Build history of the part. All positions in model axes, mm. Face numbers are marked on the shaded views. Give positions to 0.01 mm unless a question says otherwise; leave off trailing zeros. Order: outer loops, then holes, each group sorted by start corner. A loop starts at its lowest first (then second) coordinate and runs counter-clockwise, first axis right, second up. Notation, with made-up numbers: (46.5, 78) -> (62.5, 78) arc R16 cw to (62.5, 91) -> close; hole circle Ø2 at (26.5, 45). An arc over 180 degrees is marked (long way). One line per item, written item: value. Start each with the question number.
(1) Saw through at A-A on z = -31.75. Give the cut face in (x, y), plus the area to 3 significant figures.
(2) Pin check, flat tips, straight feed: pin 1 (3.5 mm diameter, centred on y = -3.37, z = 65.18, fed in from +X); pin 2 (0.5 mm diameter, centred on x = 1, y = 2, fed in from +Z); pin 3 (7 mm diameter, centred on y = 0, z = 0, fed in from +X); pin 4 (0.8 mm diameter, centred on x = 0.5, z = -20.5, fed in from -Y). Stop position of each tip, or through.
(3) Probe line 1 (Y direction, x = 1.55, z = 67); line 2 (Y direction, x = 0.2, z = -33.5); line 3 (Z direction, x = 0.9, y = 68.5). List the from-to ranges inside material, lowest first.
(4) Saw through at C-C on x = 0.8. Count the separate pieces of the cut face and the enclosed holes in it, plus the area to 3 significant figures.
(5) Two-plate mould, pull along X, no slides. Class the marked faces 1 and 2: +X half, -X half, draft (parallel to the pull), parting line (faces both ways), or undercut.
(6) Saw through at B-B on y = 44.45. Give the cut face in (x, z).
(7) Saw through at D-D on z = 16.5. Give the cut face in (x, y), plus the area to 3 significant figures.
Autodesk Inventor part; units mm, degrees
ref_plane "YZ Plane" through (0, 0, 0) normal (1, 0, 0) x (0, 1, 0)
ref_plane "XZ Plane" through (0, 0, 0) normal (0, 1, 0) x (-1, 0, 0)
ref_plane "XY Plane" through (0, 0, 0) normal (0, 0, 1) x (1, 0, 0)
sketch "main" plane through (0, 0, 0) normal (0, 0, 1) x (1, 0, 0)
  circle A0 centre (-191.7635, 49.9495) radius 2.1844
  circle A1 centre (-95.8324, -13.8772) radius 2.1
  arc A2 (-99.5462, -18.9735) -> (-92.0695, -8.7075) centre (-95.8064, -13.8415) ccw
  arc A3 (-198.1111, 49.7757) -> (-191.7635, 43.5995) centre (-191.7635, 49.9495) ccw
  line L0 (-200.5697, 139.5363) -> (-198.1111, 49.7757)
  arc A4 (-199.0195, 139.7975) -> (-92.0695, -8.7075) centre (80.274, 228.1743) ccw
  circle A5 centre (-195.1368, 115.1254) radius 2.0828
  line L1 (-191.7635, 43.5995) -> (-186.2072, 43.5995)
  arc A6 (-199.0195, 139.7975) -> (-200.5697, 139.5363) centre (-199.7762, 139.5581) ccw
  circle A7 centre (-135.2274, 18.1995) radius 2.0828
  circle A8 centre (-191.7635, 8.6745) radius 2.1844
  arc A9 (-191.7635, 15.0245) -> (-193.2141, 2.4924) centre (-191.7635, 8.6745) ccw
  line L2 (-185.4135, 15.8183) -> (-185.4135, 42.8058)
  line L3 (-191.7635, 15.0245) -> (-186.2072, 15.0245)
  arc A10 (-185.4135, 42.8058) -> (-186.2072, 43.5995) centre (-186.2072, 42.8058) ccw
  arc A11 (-186.2072, 15.0245) -> (-185.4135, 15.8183) centre (-186.2072, 15.8183) ccw
  line L4 (-193.2141, 2.4924) -> (-97.2571, -20.0236)
  point P0 (1.1251, 9.7944)
  point P1 (-200.7302, 145.398)
  dimension "d7" = 12.7
  dimension "d8" = 4.1656
  dimension "d9" = 6.35
  dimension "d11" = 0.7937
  dimension "d13" = 4.1656
  dimension "d15" = 12.7
  dimension "d16" = 0.7937
sketch "Sketch1" plane through (0, 0, 0) normal (1, 0, 0) x (0, 1, 0)
  circle A0 centre (44.45, -15.875) radius 2.0955
  circle A1 centre (0, 0) radius 2.1844
  circle A2 centre (95.9311, -63.8268) radius 2.1
  arc A3 (92.2173, -68.923) -> (99.694, -58.6571) centre (95.9571, -63.7911) ccw
  arc A4 (-6.3476, -0.1739) -> (0, -6.35) centre (0, 0) ccw
  line L0 (-8.8062, 89.5868) -> (-6.3476, -0.1739)
  arc A5 (-7.256, 89.848) -> (99.694, -58.6571) centre (272.0375, 178.2247) ccw
  circle A6 centre (-3.3733, 65.1759) radius 2.0828
  line L1 (0, -6.35) -> (5.5563, -6.35)
  arc A7 (-7.256, 89.848) -> (-8.8062, 89.5868) centre (-8.0127, 89.6085) ccw
  circle A8 centre (56.5361, -31.75) radius 2.0828
  circle A9 centre (0, -41.275) radius 2.1844
  arc A10 (0, -34.925) -> (-1.4506, -47.4571) centre (0, -41.275) ccw
  line L2 (6.35, -34.1313) -> (6.35, -7.1438)
  line L3 (0, -34.925) -> (5.5563, -34.925)
  arc A11 (6.35, -7.1438) -> (5.5563, -6.35) centre (5.5563, -7.1437) ccw
  arc A12 (5.5563, -34.925) -> (6.35, -34.1313) centre (5.5563, -34.1313) ccw
  line L4 (-1.4506, -47.4571) -> (94.5064, -69.9732)
  dimension "d18" = 4.191
extrude "Extrusion1" add sketch "Sketch1" along normal blind 1.5875
equation "\"BendRadius\" = Thickness"
equation "\"BendReliefWidth\" = Thickness"
equation "\"BendReliefDepth\" = 0.5 * Thickness"
equation "\"CornerReliefSize\" = 4 * Thickness"
equation "\"MinimumRemnant\" = 2 * Thickness"
equation "\"TransitionRadius\" = BendRadius"
equation "\"JacobiRadiusSize\" = BendRadius"
equation "\"GapSize\" = Thickness"
properties part number "ramp" material "Acetal Resin, White"
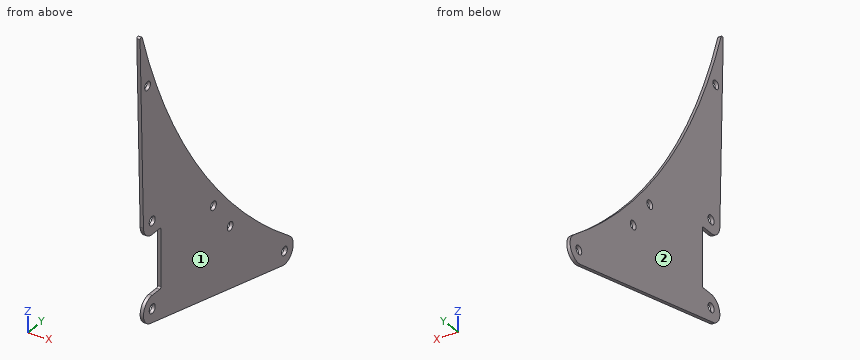
Results below:
1. outline: (0, 6.35) -> (1.59, 6.35) -> (1.59, 54.45) -> (0, 54.45) -> close; (0, 58.62) -> (1.59, 58.62) -> (1.59, 67.77) -> (0, 67.77) -> close
1. area: 90.9 mm²
2. pin 1: passes through
2. pin 2: stops at z = 65.26
2. pin 3: stops at x = 1.59
2. pin 4: stops at y = 6.35
3. line 1: y = -8.19 to -4.38, -2.37 to 1.03
3. line 2: y = 6.35 to 55.41, 57.67 to 69.58
3. line 3: z = -63.87 to -32.46
4. separate pieces: 1
4. enclosed holes: 6
4. area: 5,680 mm²
5. face 1: +X half
5. face 2: -X half
6. outline: (0, -58.23) -> (1.59, -58.23) -> (1.59, -17.97) -> (0, -17.97) -> close; (0, -13.78) -> (1.59, -13.78) -> (1.59, -6.22) -> (0, -6.22) -> close
7. outline: (0, -6.8) -> (1.59, -6.8) -> (1.59, 27.78) -> (0, 27.78) -> close
7. area: 54.9 mm²
